Input: part model. Units: mm. Frame: model coordinates. A direction names the side the tool comes from. Round coordinates to 2 decimals unless told otherwise and drop trailing zeros. Loops run counter-clockwise (first coordinate to the right, second up) from the corner with the lowest first, then second, coordinate; pieces in that order, holes last. Notation, with made-up numbers: (55, 66.25) -> (85, 66.25) arc R17 ccw to (85, 71.25) -> close; hole circle Ø4 at (-13.5, 82). An arc over 180 degrees is marked (long way). Answer as a JSON object with one key per item and string values. Group by question number.
Item 1: Set-up query: faces 1 (the flat face through (-40.5, 5, -17)), 2 (the cylindrical face through (-71.528, 114.43, -16.204)). Return all of +Z, -Z, +X, -X, +Y, -Y with unobstructed straight access to the full face (end or side cutting, diameter ignored); none if empty.
Item 2: Pin query (flat end, axial travel): pin 1 (5 mm diameter, centred on x = -91, z = -21, fed in from -Y); pin 2 (1 mm diameter, centred on x = -61.5, y = 80.5, fed in from -Z); pin 3 (1.5 mm diameter, centred on x = -73, z = -16.5, fed in from +Y). Return the tip coordinate at first contact, or that it passes through.
Item 3: Section query B-B on y = -74.5. Return loops of the section in (x, z), and give its area (3 significant figures).
Item 4: Section query A-A on x = -91. Return loops of the section in (y, z), and give its area (3 significant figures).
Item 5: Material intervals for line 1 (Y direction, x = -83, z = -7); line 2 (Y direction, x = -59.5, z = -19.5); line 3 (Z direction, x = -77, y = -60.5), sorted ascending. Write a range as [from, to].
from build123d import *

# Parameters (mm, degrees)
SKETCH004_W  = 57
SKETCH004_H  = 127
PAD002_DEPTH = 34
SKETCH005_W  = 25
SKETCH005_H  = 16
PAD003_DEPTH = 40
PAD003_TAPER = 4
SKETCH006_R  = 2.65
PAD004_DEPTH = 10
SKETCH007_R  = 6
PAD005_DEPTH = 32
PAD005_TAPER = 4


with BuildPart() as part:
    # Sketch004 → Pad002 (new body)
    with BuildSketch(Plane.XY):
        Rectangle(SKETCH004_W, SKETCH004_H)
    extrude(amount=-PAD002_DEPTH)

    # Sketch005 (on Face1 of Pad002) → Pad003 (join)
    with BuildSketch(Plane(origin=(0, 63.5, 0), x_dir=(-1, 0, 0), z_dir=(0, 1, 0))):
        with Locations((0, -17)):
            Rectangle(SKETCH005_W, SKETCH005_H)
    extrude(amount=PAD003_DEPTH, taper=PAD003_TAPER)

    # Sketch006 (on Face11 of Pad003) → Pad004 (join)
    with BuildSketch(Plane(origin=(0, 103.5, 0), x_dir=(-1, 0, 0), z_dir=(0, 1, 0))):
        with Locations((0, -17)):
            Circle(SKETCH006_R)
    extrude(amount=PAD004_DEPTH)

    # Sketch007 (on Face10 of Pad004) → Pad005 (join)
    with BuildSketch(Plane.XZ.offset(63.5)):
        with Locations((-10.5, -17)):
            Circle(SKETCH007_R)
    extrude(amount=PAD005_DEPTH, taper=PAD005_TAPER)


with BuildPart() as part_1:
    # Body002 placement: moved
    add(part.part.moved(Location((63, 6, 0))))


with BuildPart() as part_2:
    # Body003 placement: moved
    add(part_1.part.moved(Location((-132, 0, 0))))


solid = part_2.part
Solved:
{
 "1": {"face 1": "+Z, -Z, +X, +Y, -Y", "face 2": "+Y"},
 "2": {"pin 1": "y = -57.5", "pin 2": "z = -24.27", "pin 3": "y = 109.5"},
 "3": {"outline": "circle Ø9.62 at (-79.5, -17)", "area": "72.7 mm²"},
 "4": {"outline": "(-57.5, -34) -> (69.5, -34) -> (69.5, 0) -> (-57.5, 0) -> close", "area": "4,320 mm²"},
 "5": {"line 1": "[-57.5, 69.5]", "line 2": "[-57.5, 109.5]", "line 3": "[-22.22, -11.78]"}
}
